```python
from build123d import *

# Parameters (mm, degrees)
CIRPATTERN1_COUNT = 6


with BuildPart() as part:
    # Sketch1 → Revolve1 (revolve)
    with BuildSketch(Plane(origin=(0, 0, 0), x_dir=(0, 0, -1), z_dir=(1, 0, 0))):
        Polygon((19.84375, 0), (28.575, 0), (28.575, 9.525), (20.6375, 9.525), (20.6375, 15.875), (19.84375, 17.4625), align=None)
    revolve(axis=Axis((0, 73.584156028, 0), (0, -1, 0)))

    # Sketch2 → 9/32 (0.28125) Diameter Hole1 (revolve, cut)
    with BuildSketch(Plane(origin=(23.425888069, 4.7625, 16.363324637), x_dir=(0.572644782, 0, -0.819803607), z_dir=(0, 1, 0))):
        Polygon((0, 0), (0, 5.448199024), (3.571875, 3.302), (3.571875, 0), align=None)
    f_9_32_0_28125_diameter_hole1 = revolve(axis=Axis((28.631640973, 4.7625, 19.999619001), (-0.819803607, 0, -0.572644782)), mode=Mode.SUBTRACT)

    # CirPattern1: 9/32 (0.28125) Diameter Hole1 ×6 about axis
    cirpattern1_axis = Axis((0, 73.584156028, 0), (0, 1, 0))
    for i in range(1, CIRPATTERN1_COUNT):
        add(f_9_32_0_28125_diameter_hole1.rotate(cirpattern1_axis, i * 360 / CIRPATTERN1_COUNT), mode=Mode.SUBTRACT)


solid = part.part
```
Can you work these out from the model? Positions are in its coordinate system, mm. A direction names the side the tool comes from. Round coordinates to 2 decimals unless told otherwise and drop trailing zeros. Loops run counter-clockwise (first coordinate to the right, second up) from the corner with the lowest first, then second, coordinate; pieces in that order, holes last. Notation, with made-up numbers: (-35.5, 54.25) -> (14.5, 54.25) arc R25 ccw to (14.5, 86.25) -> close; hole circle Ø7 at (28.5, 64.5). An arc over 180 degrees is marked (long way). Answer in a Markdown table with one row per item.
Item 1: On a 3-axis mill with a long thin cutter (end or side, diameter ignored), from which of +Z, -Z, +X, -X, +Y, -Y can I reach the whole of each face in a straight line? I mean faces 5 (the conical face through (21.036, 4.576, -10.491)), 6 (the cylindrical face through (28.33, 4.83, 3.72)). Say none if no direction works.
Answer block:
| item | result |
|---|---|
| face 5 | none |
| face 6 | +Y, -Y |
Item 2: Suppose I cut it at B-B, the plane y = 13. List the corners of the cut face in (x, z) for me (1 decimal).
Answer block:
| item | result |
|---|---|
| outline | circle Ø41.3 at (0, 0); hole circle Ø39.7 at (0, 0) |
Item 3: If I drill on probe 1 along X at (y, z) = (4.25, 0) (3 decimals); probe 2 along Y at (x, z) = (-10, 23) (3 decimals); probe 3 along X at (y, z) = (10.75, 0), over which ranges is the centre line in solid material (lowest first)?
Answer block:
| item | result |
|---|---|
| probe 1 | -28.575 to -19.844, 19.844 to 28.575 |
| probe 2 | 0 to 9.525 |
| probe 3 | -20.64 to -19.84, 19.84 to 20.64 |
Item 4: Suppose I cut it at A-A, the plane z = 0. List the corners of the cut face in (x, y) for me (1 decimal), plus the area to 3 significant figures.
Answer block:
| item | result |
|---|---|
| outline | (-28.6, 0) -> (-19.8, 0) -> (-19.8, 17.5) -> (-20.6, 15.9) -> (-20.6, 9.5) -> (-28.6, 9.5) -> close; (19.8, 0) -> (28.6, 0) -> (28.6, 9.5) -> (20.6, 9.5) -> (20.6, 15.9) -> (19.8, 17.5) -> close |
| area | 178 mm² |
Item 5: We'd pull the mould along Y, two halves only. Please class faces 1 (the flat face through (-5.9, 0, -19.5)), 2 (the flat face through (9, 9.525, -19)), 3 (the cylindrical face through (-20.147, 12.744, 4.474)), 4 (the cylindrical face through (20.05, 4.61, 18.36)): released by +Y, released by -Y, zero draft, split by the parting line, or undercut.
Answer block:
| item | result |
|---|---|
| face 1 | released by -Y |
| face 2 | released by +Y |
| face 3 | zero draft |
| face 4 | undercut |
Item 6: Will these pins go through, and if not, where does the flat tip stop? P1, Ø10, axis at y = 11.5, z = -14.5, coming from the +X side; P2, Ø8, axis at x = 18.5, y = 13, coming from the +Z side; P3, Ø3, axis at x = -13.5, z = -9.5, coming from the +Y side; P4, Ø5, axis at x = -13, y = 14, coming from the +Z side.
Answer block:
| item | result |
|---|---|
| P1 | x = 26.8 |
| P2 | z = 23.32 |
| P3 | through |
| P4 | z = 17.77 |
